```python
from build123d import *

# Parameters (mm, degrees)
CROQUIS1_R              = 12.5
SALIENTE_EXTRUIR1_DEPTH = 5
CROQUIS2_W              = 55
CROQUIS2_H              = 5
SALIENTE_EXTRUIR2_DEPTH = 41.9


with BuildPart() as part:
    # Croquis1 → Saliente-Extruir1 (new body)
    with BuildSketch(Plane.XY):
        Polygon((0, 105), (27.5, 105), (27.5, 0), (-27.5, 0), (-27.5, 105), align=None)
        with Locations((0, 66.9)):
            Circle(CROQUIS1_R, mode=Mode.SUBTRACT)
    extrude(amount=SALIENTE_EXTRUIR1_DEPTH)

    # Croquis2 → Saliente-Extruir2 (add)
    with BuildSketch(Plane.XY.offset(5)):
        with Locations((0, 2.5)):
            Rectangle(CROQUIS2_W, CROQUIS2_H)
    extrude(amount=SALIENTE_EXTRUIR2_DEPTH)


solid = part.part
```
Read the model definition and answer for the solid it produces. Units are mm, in the model's axes. A direction names the side the tool comes from. Round coordinates to 2 decimals unless told otherwise and drop trailing zeros. Write each loop counter-clockwise with the first axis right and the second up, starting at its lowest first coordinate (ties: lowest second). Pieces come first, ordered by that corner, then holes. Notation, with made-up numbers: (63.25, -23.75) - (115.25, -23.75) arc R17 ccw to (115.25, -11.75) - close; hole circle Ø6 at (72, 85.25). An arc over 180 degrees is marked (long way). Use CSV: the item, a comma, the result in double quotes.
Q1. Find section D-D, the plane z = 9. Write down the section's boundary in (x, y), then the cut area to 3 significant figures.
Values:
outline,"(-27.5, 0) - (27.5, 0) - (27.5, 5) - (-27.5, 5) - close"
area,"275 mm²"
Q2. Determine the mould class of faces 1 (the flat face through (27.5, 41, 4)), 2 (the flat face through (0, 5, 26)), 3 (the cylindrical face through (-1.627, 79.294, 2.465)) for opening direction X: +X half, -X half, draft (parallel to the pull), parting line (faces both ways), or undercut.
Values:
face 1,"+X half"
face 2,"draft"
face 3,"undercut"
Q3. Find section C-C, the plane x = 21. Write down the section's boundary in (y, z).
Values:
outline,"(0, 0) - (105, 0) - (105, 5) - (5, 5) - (5, 46.9) - (0, 46.9) - close"
Q4. A tool of negligible diameter and unlimited length cuts with its end or side. For faces 4 (the flat face through (-27.5, 41, 4)), 5 (the flat face through (6.5, 55.7, 5)), from which of +Z, -Z, +X, -X, +Y, -Y can it reach the whole face along a straight path? Write none if from no direction.
Values:
face 4,"+Z, -Z, -X, +Y, -Y"
face 5,"+Z, +X, -X, +Y"
Q5. Find section A-A, the plane y = 66.9. Write down the section's boundary in (x, z), then the cut area to 3 significant figures.
Values:
outline,"(-27.5, 0) - (-12.5, 0) - (-12.5, 5) - (-27.5, 5) - close; (12.5, 0) - (27.5, 0) - (27.5, 5) - (12.5, 5) - close"
area,"150 mm²"
Q6. This flat-tipped pin is pushed along its axis until it touches: pin 1 Ø3 at (x, z) = (-12.5, 12.5) entering from +Y. Where does it stop, or does it pass through?
Values:
pin 1,"stops at y = 5"
Q7. Find section B-B, the plane x = 0. Write down the section's boundary in (y, z), then the cut area to 4 significant figures.
Values:
outline,"(0, 0) - (54.4, 0) - (54.4, 5) - (5, 5) - (5, 46.9) - (0, 46.9) - close; (79.4, 0) - (105, 0) - (105, 5) - (79.4, 5) - close"
area,"609.5 mm²"
Q8. Straight lines are drawn through the part: line 1 along Y through (x, z) = (0, 2); line 2 along Y through (x, z) = (23.5, 5.5). For each, find the intervals that lie inside material, in ascending order.
Values:
line 1,"y = 0 to 54.4, 79.4 to 105"
line 2,"y = 0 to 5"
